Geometry check sheet. Reference: the model listing, model coordinates, mm. Face numbers are marked on the shaded views. A direction names the side the tool comes from. Coordinates: 2 decimals unless noted, no trailing zeros. Loops run counter-clockwise (first coordinate to the right, second up) from the corner with the lowest first, then second, coordinate; pieces in that order, holes last.
from build123d import *

# Parameters (mm, degrees)
F1_DEPTH = 150
F2_W     = 100
F2_H     = 297.664444
F2_H_2   = 25
F3_DEPTH = 10000
F5_DEPTH = 10000


with BuildPart() as f1:
    # F0 (on Front) → F1 (new body)
    with BuildSketch(Plane.XZ):
        with BuildLine():
            Line((-250, -25), (250, -25))
            Line((250, -25), (250, 25))
            ThreePointArc((250, 25), (0, 275), (-250, 25))
            Line((-250, 25), (-250, -25))
        make_face()
    extrude(amount=-F1_DEPTH)

    # F2 (on face) → F3 (cut)
    with BuildSketch(Plane(origin=(-250, 0, 0), x_dir=(0, -1, 0), z_dir=(-1, 0, 0))):
        with Locations((-75, 173.832222)):
            Rectangle(F2_W, F2_H)
        with Locations((-75, 12.5)):
            Rectangle(F2_W, F2_H_2)
    extrude(amount=-F3_DEPTH, mode=Mode.SUBTRACT)

    # F4 (on face) → F5 (cut)
    with BuildSketch(Plane(origin=(0, 150, 0), x_dir=(-1, 0, 0), z_dir=(0, 1, 0))):
        with BuildLine():
            Line((-233.881947, 0), (-50.46213, 0))
            Line((-50.46213, 0), (-222.4755, 88.46351))
            ThreePointArc((-222.4755, 88.46351), (-232.40746, 44.777007), (-233.881947, 0))
        make_face()
        with BuildLine():
            Line((-37.298094, 53.475399), (-107.561018, 223.502855))
            ThreePointArc((-107.561018, 223.502855), (-159.267001, 187.027318), (-199.387616, 138.095635))
            Line((-199.387616, 138.095635), (-37.298094, 53.475399))
        make_face()
        with BuildLine():
            Line((0, 67.517042), (46.411204, 245.636359))
            ThreePointArc((46.411204, 245.636359), (-3.315529, 250.011517), (-52.846596, 243.801574))
            Line((-52.846596, 243.801574), (0, 67.517042))
        make_face()
        with BuildLine():
            Line((34.665316, 50.842591), (191.731855, 152.647342))
            ThreePointArc((191.731855, 152.647342), (152.861228, 194.537882), (105.04086, 225.826144))
            Line((105.04086, 225.826144), (34.665316, 50.842591))
        make_face()
        with BuildLine():
            ThreePointArc((235.951228, 0), (233.540018, 51.316805), (220.052612, 100.88815))
            Line((220.052612, 100.88815), (38.175728, 0))
            Line((38.175728, 0), (235.951228, 0))
        make_face()
    extrude(amount=-F5_DEPTH, mode=Mode.SUBTRACT)


solid = f1.part
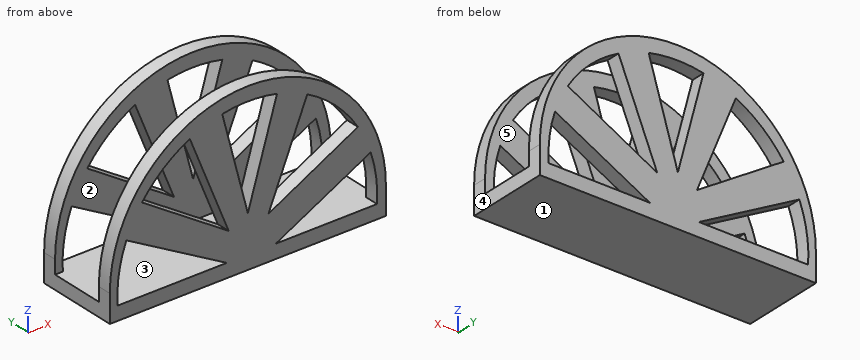
1) Material ranges on probe 1 along Y at (x, z) = (-62, 174); probe 2 along Z at (x, y) = (122, 19); probe 3 along Z at (x, y) = (106, 7.5), recorded low to high.
Data:
probe 1: y = 0 to 25, 125 to 150
probe 2: z = -25 to 0, 36.79 to 97.69, 215.34 to 243.21
probe 3: z = -25 to 0, 28.56 to 89.34, 219.73 to 251.42
2) Section check B-B on x = 208. Record the cut outline in (y, z), and give its area (3 significant figures).
Data:
outline: (0, -25) - (150, -25) - (150, 0) - (0, 0) - close; (0, 81.02) - (25, 81.02) - (25, 163.69) - (0, 163.69) - close; (125, 81.02) - (150, 81.02) - (150, 163.69) - (125, 163.69) - close
area: 7,880 mm2
3) Access from +Z, -Z, +X, -X, +Y, -Y to the whole of each face (thin tool, end or side, straight path). Record for the marked faces 1 and 2.
Data:
face 1: -Z, +X, -X, +Y, -Y
face 2: +Z, +X, -X
4) Section check C-C on z = 162.5. Count the separate pieces of the cut face and the enclosed holes in it, and give its area (3 significant figures).
Data:
separate pieces: 8
enclosed holes: 0
area: 8,000 mm2
5) Section check D-D on y = 15.5. Record the cut outline in (x, z).
Data:
outline: (-250, -25) - (250, -25) - (250, 25) arc R250 ccw to (-250, 25) - close; hole (-235.95, 0) - (-38.18, 0) - (-220.05, 100.89) arc R235.37 ccw to start; hole (-191.73, 152.65) - (-34.67, 50.84) - (-105.04, 225.83) arc R235.37 ccw to start; hole (-46.41, 245.64) - (0, 67.52) - (52.85, 243.8) arc R235.37 ccw to start; hole (37.3, 53.48) - (199.39, 138.1) arc R235.37 ccw to (107.56, 223.5) - close; hole (50.46, 0) - (233.88, 0) arc R235.37 ccw to (222.48, 88.46) - close
6) Mould release check, pull along X, two halves, no side actions. Record for the marked faces 3, 4 and 5: +X half, -X half, draft (parallel to the pull), parting line (faces both ways), or undercut.
Data:
face 3: undercut
face 4: +X half
face 5: draft
7) Section check A-A on z = 32.5. Record the cut outline in (x, y).
Data:
outline: (-249.89, 0) - (-235.73, 0) - (-235.73, 25) - (-249.89, 25) - close; (-249.89, 125) - (-235.73, 125) - (-235.73, 150) - (-249.89, 150) - close; (-96.77, 0) - (113.66, 0) - (113.66, 25) - (-96.77, 25) - close; (-96.77, 125) - (113.66, 125) - (113.66, 150) - (-96.77, 150) - close; (233.66, 0) - (249.89, 0) - (249.89, 25) - (233.66, 25) - close; (233.66, 125) - (249.89, 125) - (249.89, 150) - (233.66, 150) - close
